Input: part model. Units: mm. Frame: model coordinates. A direction names the side the tool comes from. Round coordinates to 2 decimals unless told otherwise and drop trailing zeros. Loops run counter-clockwise (first coordinate to the right, second up) from the corner with the lowest first, then second, coordinate; pieces in that order, holes last. Notation, with made-up numbers: (30.25, -35.5) -> (76.25, -35.5) arc R35 ccw to (76.25, -2.5) -> close; hole circle Ø3 at (40.25, 84.5). An arc over 180 degrees is marked (long way). Answer as a JSON object with one key per item and string values. Group by question number.
Item 1: Section query A-A on y = 3.5. Return loops of the section in (x, z).
Item 2: Section query D-D on y = -11. Return loops of the section in (x, z).
Item 3: Section query C-C on z = 1. Return loops of the section in (x, y) (3 decimals).
Item 4: Draft query along Y for faces 4 (the flat face through (20.7, -24.82, -15.34)), 5 (the cylindrical face through (69.768, 1.769, -18.961)), 6 (the flat face through (29, 0, 0)), 7 (the cylindrical face through (-15.12, -11.59, -0.36)). Return one class per face: released by +Y, released by -Y, zero draft, split by the parting line, or undercut.
Item 5: Set-up query: faces 1 (the cylindrical face through (31.75, 0.05, -6.26)), 2 (the cylindrical face through (59.6, -3.65, -18.96)), 3 (the flat face through (5.3, 27.8, 0)). Return all of +Z, -Z, +X, -X, +Y, -Y with unobstructed straight access to the full face (end or side cutting, diameter ignored); none if empty.
Item 6: Section query B-B on x = 53. Return loops of the section in (y, z), and give its area (3 significant figures).
Item 7: Pin query (flat end, axial travel): pin 1 (17 mm diameter, centred on x = 50.8, y = 0, fed in from +Z); pin 2 (1 mm diameter, centred on y = -1, z = 13.5, fed in from -X); pin 3 (19 mm diameter, centred on x = 44.5, y = 1.5, fed in from +Z); pin 4 (5 mm diameter, centred on x = 39.5, z = -5, fed in from -Y). Return the tip coordinate at first contact, or that it passes through.
Item 8: Material intervals for line 1 (X direction, y = 6, z = -21.5); line 2 (Y direction, x = 50.8, z = -16.5) (3 decimals); line 3 (Y direction, x = 16, z = -17), sorted ascending. Write a range as [from, to].
from build123d import *

# Parameters (mm, degrees)
F0_R        = 19.05
F0_R_2      = 9.525
F1_DEPTH    = 25.4
F2_DEPTH    = 25.4
F3_DEPTH    = 12.7
F4_T1_DEPTH = 57.2245179891
F4_T3_DEPTH = 67.6926131403


# Not quite as in the source:
# - a fillet or chamfer that OpenCascade refuses, or shapes differently, is made with other operations: its cross-section is extruded or revolved along the edge and cut away or added


with BuildPart() as f1:
    # F0 (on Top) → F1 (new body)
    with BuildSketch(Plane.XY):
        with BuildLine():
            Line((10.5539222721, 26.5545730464), (0, 28.575))
            ThreePointArc((0, 28.575), (-28.575, 0), (0, -28.575))
            Line((0, -28.575), (10.035773719, -26.7546981082))
            ThreePointArc((10.035773719, -26.7546981082), (23.4872610048, -16.2751096921), (28.575, 0))
            ThreePointArc((28.575, 0), (23.644332872, 16.046063319), (10.5539222721, 26.5545730464))
        make_face()
        Circle(F0_R, mode=Mode.SUBTRACT)
        with BuildLine():
            Line((49.8728171001, 19.0274231537), (10.5539222721, 26.5545730464))
            ThreePointArc((10.5539222721, 26.5545730464), (23.644332872, 16.046063319), (28.575, 0))
            ThreePointArc((28.575, 0), (23.4872610048, -16.2751096921), (10.035773719, -26.7546981082))
            Line((10.035773719, -26.7546981082), (54.1998407335, -18.7441613039))
            ThreePointArc((54.1998407335, -18.7441613039), (31.8737838621, -2.1681426844), (49.8728171001, 19.0274231537))
        make_face()
        with BuildLine():
            ThreePointArc((69.85, 0), (63.9384867043, 13.7942983555), (49.8728171001, 19.0274231537))
            ThreePointArc((49.8728171001, 19.0274231537), (31.8737838621, -2.1681426844), (54.1998407335, -18.7441613039))
            ThreePointArc((54.1998407335, -18.7441613039), (65.4230890371, -12.2093311452), (69.85, 0))
        make_face()
        with Locations((50.8, 0)):
            Circle(F0_R_2, mode=Mode.SUBTRACT)
    extrude(amount=-F1_DEPTH)

    # F0 (on Top) → F2 (join)
    with BuildSketch(Plane.XY):
        with BuildLine():
            Line((10.5539222721, 26.5545730464), (0, 28.575))
            ThreePointArc((0, 28.575), (-28.575, 0), (0, -28.575))
            Line((0, -28.575), (10.035773719, -26.7546981082))
            ThreePointArc((10.035773719, -26.7546981082), (23.4872610048, -16.2751096921), (28.575, 0))
            ThreePointArc((28.575, 0), (23.644332872, 16.046063319), (10.5539222721, 26.5545730464))
        make_face()
        Circle(F0_R, mode=Mode.SUBTRACT)
        with BuildLine():
            Line((10.035773719, -26.7546981082), (0, -28.575))
            ThreePointArc((0, -28.575), (5.0997611002, -28.1162419559), (10.035773719, -26.7546981082))
        make_face()
        with BuildLine():
            ThreePointArc((10.5539222721, 26.5545730464), (5.3727879262, 28.0653482947), (0, 28.575))
            Line((0, 28.575), (10.5539222721, 26.5545730464))
        make_face()
    extrude(amount=F2_DEPTH)

    # F0 (on Top) → F3 (cut)
    with BuildSketch(Plane.XY):
        with BuildLine():
            ThreePointArc((69.85, 0), (63.9384867043, 13.7942983555), (49.8728171001, 19.0274231537))
            ThreePointArc((49.8728171001, 19.0274231537), (31.8737838621, -2.1681426844), (54.1998407335, -18.7441613039))
            ThreePointArc((54.1998407335, -18.7441613039), (65.4230890371, -12.2093311452), (69.85, 0))
        make_face()
        with Locations((50.8, 0)):
            Circle(F0_R_2, mode=Mode.SUBTRACT)
    extrude(amount=-F3_DEPTH, mode=Mode.SUBTRACT)

    # F4: fillet of radius 6.35 on 3 edges, made by hand

    # F4_s2 → F4_t1 (cut)
    with BuildSketch(Plane.XY.offset(-12.7)):
        with BuildLine():
            ThreePointArc((32.3806581498, 22.376095667), (37.1591875386, 18.2961908719), (36.0900289579, 12.1045137012))
            ThreePointArc((36.0900289579, 12.1045137012), (42.2494552996, 17.0232395662), (49.8728171001, 19.0274231537))
            Line((49.8728171001, 19.0274231537), (32.3806581498, 22.376095667))
        make_face()
    extrude(amount=F4_T1_DEPTH, mode=Mode.SUBTRACT)

    # F4_s4 → F4_t3 (cut)
    with BuildSketch(Plane.XY.offset(-12.7)):
        with BuildLine():
            ThreePointArc((32.5559475844, -22.6699592292), (37.4002807494, -18.5644828639), (36.2670005049, -12.3164290959))
            ThreePointArc((36.2670005049, -12.3164290959), (44.372267792, -17.9328402285), (54.1998407335, -18.7441613039))
            Line((54.1998407335, -18.7441613039), (32.5559475844, -22.6699592292))
        make_face()
    extrude(amount=F4_T3_DEPTH, mode=Mode.SUBTRACT)


solid = f1.part
Solved:
{
 "1": {"outline": "(-28.36, -25.4) -> (-18.73, -25.4) -> (-18.73, 25.4) -> (-28.36, 25.4) -> close; (18.73, -25.4) -> (41.94, -25.4) -> (41.94, -12.7) -> (32.07, -12.7) -> (32.07, 0) -> (28.36, 0) -> (28.36, 25.4) -> (18.73, 25.4) -> close; (59.66, -25.4) -> (69.53, -25.4) -> (69.53, -12.7) -> (59.66, -12.7) -> close"},
 "2": {"outline": "(-26.37, -25.4) -> (-15.55, -25.4) -> (-15.55, 25.4) -> (-26.37, 25.4) -> close; (15.55, -25.4) -> (66.35, -25.4) -> (66.35, -12.7) -> (35.25, -12.7) -> (35.25, 0) -> (26.37, 0) -> (26.37, 25.4) -> (15.55, 25.4) -> close"},
 "3": {"outline": "circle Ø57.15 at (0, 0); hole circle Ø38.1 at (0, 0)"},
 "4": {"face 4": "released by -Y", "face 5": "split by the parting line", "face 6": "zero draft", "face 7": "undercut"},
 "5": {"face 1": "+Z, +X", "face 2": "+Z, -Z", "face 3": "-Z, +X, +Y"},
 "6": {"outline": "(-18.96, -25.4) -> (-9.27, -25.4) -> (-9.27, -12.7) -> (-18.96, -12.7) -> close; (9.27, -25.4) -> (18.92, -25.4) -> (18.92, -12.7) -> (9.27, -12.7) -> close", "area": "246 mm²"},
 "7": {"pin 1": "through", "pin 2": "x = -28.57", "pin 3": "z = -12.7", "pin 4": "y = -19.46"},
 "8": {"line 1": "[-27.94, -18.08], [18.08, 43.4], [58.2, 68.88]", "line 2": "[-19.361, -9.525], [9.525, 19.05]", "line 3": "[-25.67, -10.34], [10.34, 25.51]"}
}
